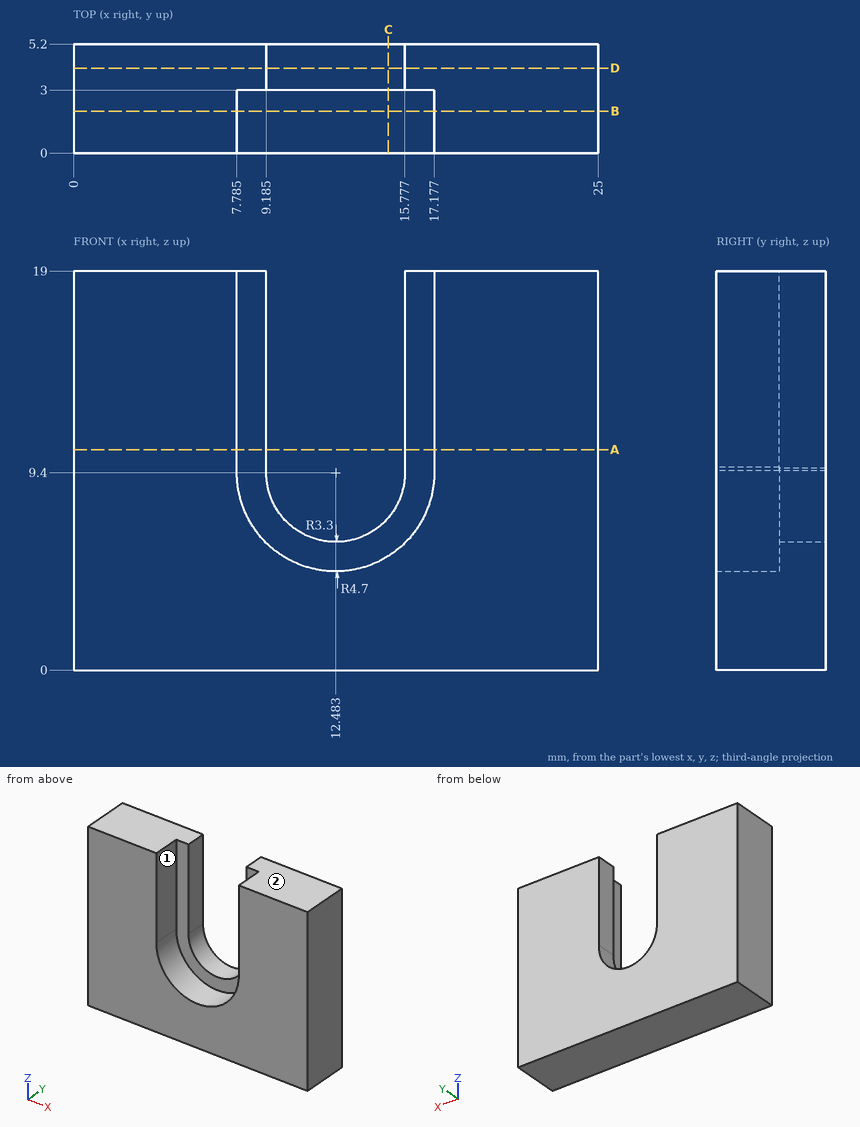
The drawing under review shows one solid part. Ordinate dimensions are in mm from its lowest x, y, z. A direction names the side the tool comes from. Coordinates: 2 decimals unless noted, no trailing zeros. Loops run counter-clockwise (first coordinate to the right, second up) from the corner with the lowest first, then second, coordinate; pieces in that order, holes last. Notation, with made-up numbers: (2.5, 55) - (24.5, 55) arc R9 cw to (24.5, 70) - close; hole circle Ø10 at (-22, -23). An arc over 180 degrees is marked (long way). Return JSON: item names as keys, results as strings.
Item 1: For line 1 (X direction, y = 1.5, z = 15.75) (1 decimal); line 2 (X direction, y = 4.9, z = 16.5) (1 decimal); line 3 (Z direction, x = 12.5, y = 3.65), list the stretches that pass through material, from the lowest coordinate up.
Determined:
{"line 1": "x = 0 to 7.8, 17.2 to 25", "line 2": "x = 0 to 9.2, 15.8 to 25", "line 3": "z = 0 to 6.1"}
Item 2: Take a section at D-D (y = 4.05). Give the boundary of the cut face in (x, z) (1 decimal).
Determined:
{"outline": "(0, 0) - (25, 0) - (25, 19) - (15.8, 19) - (15.8, 9.6) arc R3.3 cw (long way) to (9.2, 9.5) - (9.2, 19) - (0, 19) - close"}
Item 3: Take a section at B-B (y = 2). Give the boundary of the cut face in (x, z) (1 decimal), then the cut area to 3 significant figures.
Determined:
{"outline": "(0, 0) - (25, 0) - (25, 19) - (17.2, 19) - (17.2, 9.7) arc R4.7 cw (long way) to (7.8, 9.5) - (7.8, 19) - (0, 19) - close", "area": "350 mm2"}
Item 4: For the marked faces 1 and 2, list the 3-axis set-ups (+Z, -Z, +X, -X, +Y, -Y) from which the entire face can be reached by the end or side of a thin tool; tool diameter is ignored.
Determined:
{"face 1": "+Z, -Y", "face 2": "+Z, +X, -X, +Y, -Y"}
Item 5: Take a section at A-A (z = 10.5). Give the boundary of the cut face in (x, y) (1 decimal).
Determined:
{"outline": "(0, 0) - (7.8, 0) - (7.8, 3) - (9.2, 3) - (9.2, 5.2) - (0, 5.2) - close; (15.8, 3) - (17.2, 3) - (17.2, 0) - (25, 0) - (25, 5.2) - (15.8, 5.2) - close"}
Item 6: Take a section at C-C (x = 15). Give the boundary of the cut face in (y, z) (1 decimal).
Determined:
{"outline": "(0, 0) - (5.2, 0) - (5.2, 7.3) - (3, 7.3) - (3, 5.4) - (0, 5.4) - close"}
